Answer from the drawing. Dimensions are ordinates in mm from the lowest x, y and z of the part. Coordinates: 2 decimals unless noted, no trailing zeros. Order: outer loops, then holes, each group sorted by start corner. A loop starts at its lowest first (then second) coordinate and runs counter-clockwise, first axis right, second up.
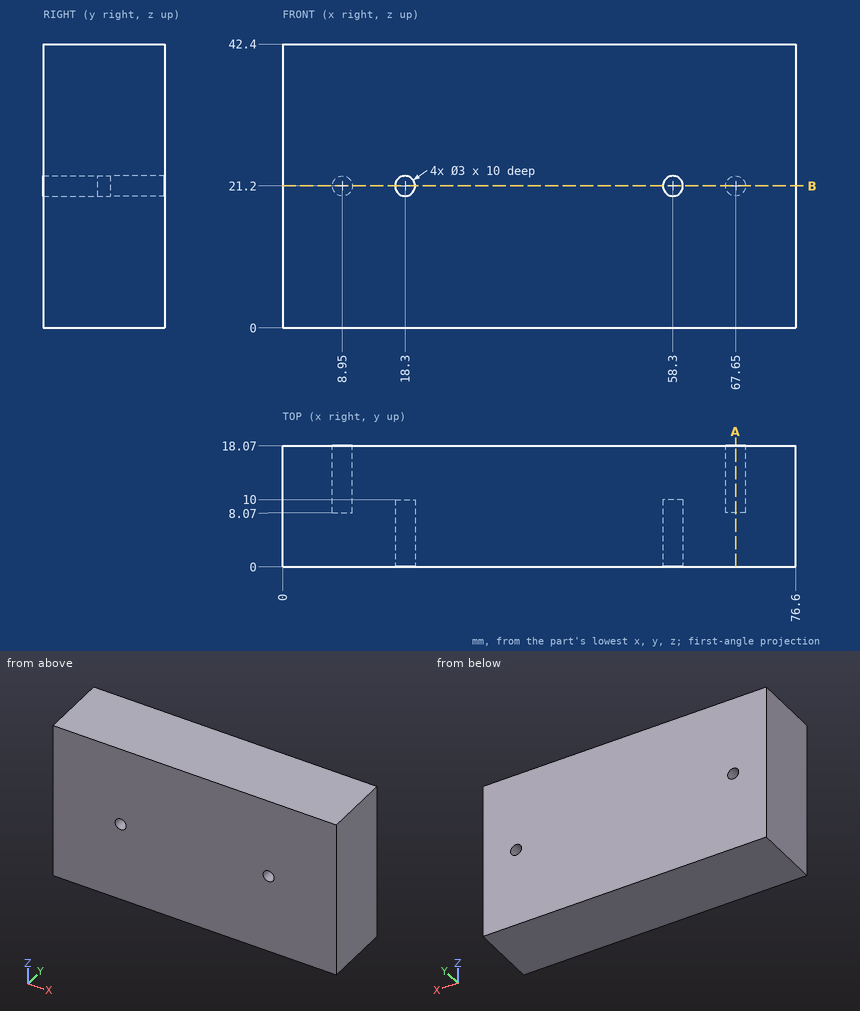
1. A flat-ended cylindrical pin translates along its axis: pin 1 (2.5 mm diameter, centred on x = 67.65, z = 21.2, fed in from +Y). Find the tip coordinate at first contact, or state that the pin passes through.
2. The part is cut by section B-B (z = 21.2). Determine the outline of the cut face in (x, y).
3. Consider probe 1 along X at (y, z) = (12.25, 21.2); probe 2 along X at (y, z) = (5.5, 21.2); probe 3 along Z at (x, y) = (58.5, 1.75). Determine where each line is inside the solid, lowest interval first.
4. The part is cut by section A-A (x = 67.65). Determine the outline of the cut face in (y, z).
Worked out:
1. pin 1: stops at y = 8.07
2. outline: (0, 0) - (16.8, 0) - (16.8, 10) - (19.8, 10) - (19.8, 0) - (56.8, 0) - (56.8, 10) - (59.8, 10) - (59.8, 0) - (76.6, 0) - (76.6, 18.07) - (69.15, 18.07) - (69.15, 8.07) - (66.15, 8.07) - (66.15, 18.07) - (10.45, 18.07) - (10.45, 8.07) - (7.45, 8.07) - (7.45, 18.07) - (0, 18.07) - close
3. probe 1: x = 0 to 7.45, 10.45 to 66.15, 69.15 to 76.6
3. probe 2: x = 0 to 16.8, 19.8 to 56.8, 59.8 to 76.6
3. probe 3: z = 0 to 19.71, 22.69 to 42.4
4. outline: (0, 0) - (18.07, 0) - (18.07, 19.7) - (8.07, 19.7) - (8.07, 22.7) - (18.07, 22.7) - (18.07, 42.4) - (0, 42.4) - close
